from build123d import *

# Parameters (mm, degrees)
SKETCH034_W   = 90
SKETCH034_H   = 140
SKETCH034_R   = 2.75
SKETCH034_R_2 = 3.5
SKETCH034_W_2 = 61.5
SKETCH034_H_2 = 14.2
PAD016_DEPTH  = 3
SKETCH033_W   = 85
SKETCH033_H   = 120
SKETCH033_W_2 = 82
SKETCH033_H_2 = 117
PAD017_DEPTH  = 5
SKETCH035_W   = 74
SKETCH035_H   = 85
SKETCH035_W_2 = 61.5
SKETCH035_H_2 = 14.2
PAD018_DEPTH  = 5
FILLET013_R   = 5
FILLET015_R   = 0.5


with BuildPart() as part:
    # Sketch034 → Pad016 (new body)
    with BuildSketch(Plane.XY):
        Rectangle(SKETCH034_W, SKETCH034_H)
        with Locations((-39, 65)):
            Circle(SKETCH034_R, mode=Mode.SUBTRACT)
        with Locations((39, 65)):
            Circle(SKETCH034_R, mode=Mode.SUBTRACT)
        with Locations((39, -65)):
            Circle(SKETCH034_R, mode=Mode.SUBTRACT)
        with Locations((-39, -65)):
            Circle(SKETCH034_R, mode=Mode.SUBTRACT)
        with Locations((-29.5, -46)):
            Circle(SKETCH034_R_2, mode=Mode.SUBTRACT)
        with Locations((0, -46)):
            Circle(SKETCH034_R_2, mode=Mode.SUBTRACT)
        with Locations((29.5, -46)):
            Circle(SKETCH034_R_2, mode=Mode.SUBTRACT)
        with Locations((1.85, 49.25)):
            Rectangle(SKETCH034_W_2, SKETCH034_H_2, mode=Mode.SUBTRACT)
        with Locations((1.85, 27.25)):
            Rectangle(SKETCH034_W_2, SKETCH034_H_2, mode=Mode.SUBTRACT)
        with Locations((1.85, 5.25)):
            Rectangle(SKETCH034_W_2, SKETCH034_H_2, mode=Mode.SUBTRACT)
        with Locations((1.85, -16.75)):
            Rectangle(SKETCH034_W_2, SKETCH034_H_2, mode=Mode.SUBTRACT)
    extrude(amount=PAD016_DEPTH)

    # Sketch033 (on Face28 of Pad016) → Pad017 (join)
    with BuildSketch(Plane(origin=(0, 0, 0), x_dir=(1, 0, 0), z_dir=(0, 0, -1))):
        Rectangle(SKETCH033_W, SKETCH033_H)
        Rectangle(SKETCH033_W_2, SKETCH033_H_2, mode=Mode.SUBTRACT)
    extrude(amount=PAD017_DEPTH)

    # Sketch035 (on Face35 of Pad017) → Pad018 (join)
    with BuildSketch(Plane(origin=(0, 0, 0), x_dir=(1, 0, 0), z_dir=(0, 0, -1))):
        with Locations((2, -16)):
            Rectangle(SKETCH035_W, SKETCH035_H)
        with Locations((1.85, -49.25)):
            Rectangle(SKETCH035_W_2, SKETCH035_H_2, mode=Mode.SUBTRACT)
        with Locations((1.85, 16.75)):
            Rectangle(SKETCH035_W_2, SKETCH035_H_2, mode=Mode.SUBTRACT)
        with Locations((1.85, -27.25)):
            Rectangle(SKETCH035_W_2, SKETCH035_H_2, mode=Mode.SUBTRACT)
        with Locations((1.85, -5.25)):
            Rectangle(SKETCH035_W_2, SKETCH035_H_2, mode=Mode.SUBTRACT)
    extrude(amount=PAD018_DEPTH)

    # Fillet013
    fillet013_edges = [part.edges().sort_by_distance(p)[0] for p in [
        (45, -70, 1.5),
        (-45, -70, 1.5),
        (-45, 70, 1.5),
        (45, 70, 1.5),
    ]]
    fillet(fillet013_edges, radius=FILLET013_R)

    # Fillet015
    fillet015_edges = [part.edges().sort_by_distance(p)[0] for p in [
        (1.85, 56.35, -5),
        (32.6, 49.25, -5),
        (-28.9, 49.25, -5),
        (1.85, 42.15, -5),
        (1.85, -9.65, -5),
        (32.6, -16.75, -5),
        (1.85, -23.85, -5),
        (-28.9, -16.75, -5),
        (1.85, 12.35, -5),
        (32.6, 5.25, -5),
        (1.85, -1.85, -5),
        (-28.9, 5.25, -5),
        (1.85, 34.35, -5),
        (-28.9, 27.25, -5),
        (1.85, 20.15, -5),
        (32.6, 27.25, -5),
    ]]
    fillet(fillet015_edges, radius=FILLET015_R)


solid = part.part
For this review, take the finished solid that the model builds, in its own axes (mm). A direction names the side the tool comes from. Give positions to 0.01 mm unless a question says otherwise; leave off trailing zeros. Loops run counter-clockwise (first coordinate to the right, second up) from the corner with the lowest first, then second, coordinate; pieces in that order, holes last. Notation, with made-up numbers: M 49,-3.75 L 102,-3.75 A21 ccw 102,11.25 Z; hole C 5,28 d2. An arc over 180 degrees is marked long. Put each result on its own line as item: value. Start each with the question number.
(1) For pin 1 (1.5 mm diameter, centred on y = 6, z = -3, fed in from +X); pin 2 (2 mm diameter, centred on y = 27.5, z = -1.5, fed in from -X); pin 3 (4 mm diameter, centred on x = -15, y = -37.5, fed in from -Z); pin 4 (4 mm diameter, centred on x = 29.5, y = -46, fed in from +Z) (3 decimals), all flat-tipped, find the tip position at first contact; note any pin that passes through.
(2) Add section A-A, the plane y = -18. Write out the cut boundary in (x, z), then the cut area to 3 significant figures.
(3) Wall thickness on L1, parallel to Y at x = 39, z = 2.4; L2, parallel to Y at x = 0, z = 1; L3, parallel to X at y = 23, z = -3.5: over which ranges is each line inside the solid? List them lowest first.
(4) Add section C-C, the plane y = -46. Write out the cut boundary in (x, z), then the cut area to 3 significant figures.
(5) Add section B-B, the plane z = 1.25. Give the number of separate pieces and of enclosed holes in the cut face, then the cut area to 3 significant figures.
(6) Machinability: for faces 1 (the flat face through (-45, -1, 1)), 2 (the flat face through (41, 1, -2)), 3 (the flat face through (1, -9.65, -1)), which of the approach directions +Z, -Z, +X, -X, +Y, -Y give a long, thin tool a straight path to every point of the face, cutting with its end or side? Answer none if there is none.
(7) The part is to be moulded in two halves that separate along Y. For faces 4 (the cylindrical face through (36.973, -63.141, 1.479)), 5 (the flat face through (45, -1, 1)), 6 (the flat face through (32.6, 27, -1)), 7 (the cylindrical face through (-43, 69, 2)), say which applies: +Y half, -Y half, draft (parallel to the pull), parting line (faces both ways), or undercut.
Result:
1. pin 1: stops at x = 42.5
1. pin 2: stops at x = -42.5
1. pin 3: stops at z = 0
1. pin 4: passes through
2. outline: M -45,0 L -42.5,0 L -42.5,-5 L -41,-5 L -41,0 L -35,0 L -35,-5 L -29.4,-5 A0.5 ccw -28.9,-4.5 L -28.9,3 L -45,3 Z; M 32.6,-4.5 A0.5 ccw 33.1,-5 L 39,-5 L 39,0 L 41,0 L 41,-5 L 42.5,-5 L 42.5,0 L 45,0 L 45,3 L 32.6,3 Z
2. area: 163 mm^2
3. L1: y = -70 to -67.75, -62.25 to 62.25, 67.75 to 70
3. L2: y = -70 to -49.5, -42.5 to -23.85, -9.65 to -1.85, 12.35 to 20.15, 34.35 to 42.15, 56.35 to 70
3. L3: x = -42.5 to -41, -35 to -28.9, 32.6 to 39, 41 to 42.5
4. outline: M -45,0 L -42.5,0 L -42.5,-5 L -41,-5 L -41,0 L -33,0 L -33,3 L -45,3 Z; M -26,0 L -3.5,0 L -3.5,3 L -26,3 Z; M 3.5,0 L 26,0 L 26,3 L 3.5,3 Z; M 33,0 L 41,0 L 41,-5 L 42.5,-5 L 42.5,0 L 45,0 L 45,3 L 33,3 Z
4. area: 222 mm^2
5. separate pieces: 1
5. enclosed holes: 11
5. area: 8,870 mm^2
6. face 1: +Z, -Z, -X, +Y, -Y
6. face 2: -Z
6. face 3: +Z, -Z
7. face 4: undercut
7. face 5: draft
7. face 6: undercut
7. face 7: +Y half
